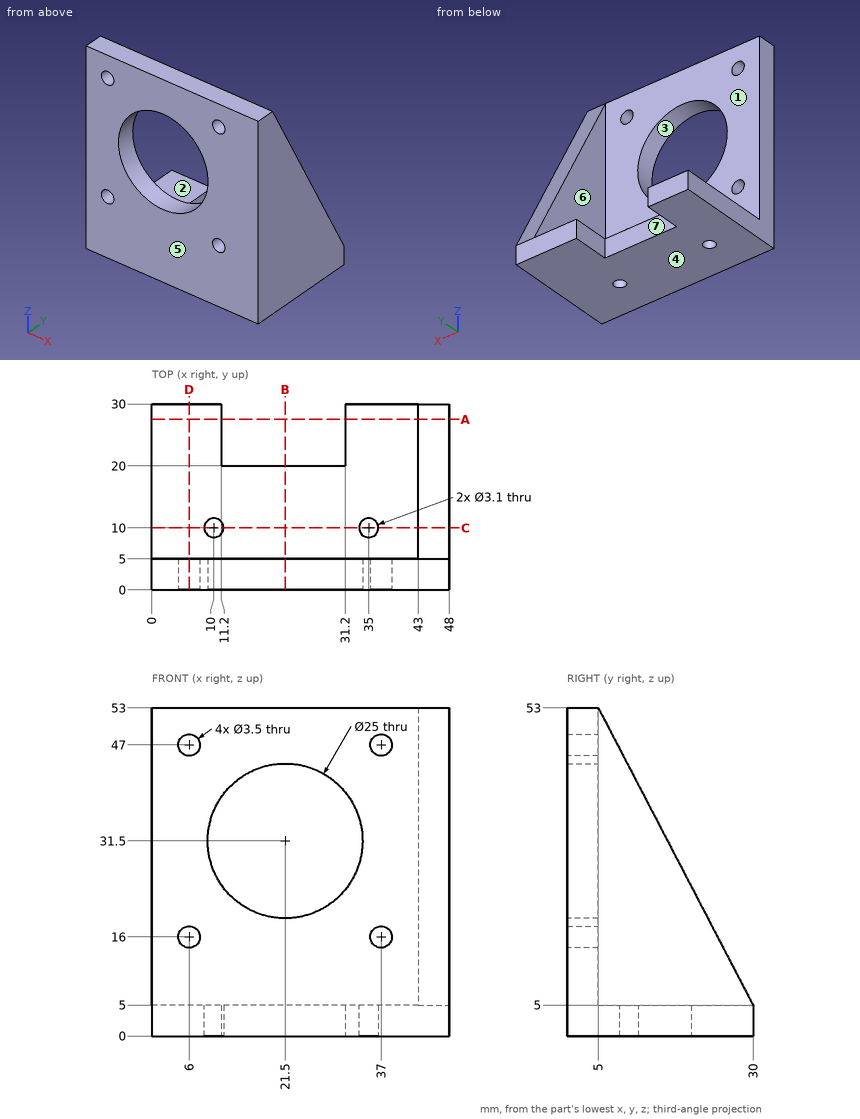
Input: dimensioned drawing with shaded views. Units: mm. Origin: part minimum x, y, z. A direction names the side the tool comes from. Coordinates: 2 decimals unless noted, no trailing zeros. Loops run counter-clockwise (first coordinate to the right, second up) from the corner with the lowest first, then second, coordinate; pieces in that order, holes last.
Q1. Section C-C, the plane y = 10. Return the cut outline in (x, z), and give its area (3 significant figures).
Results are:
outline: (0, 0) - (8.45, 0) - (8.45, 5) - (0, 5) - close; (11.55, 0) - (33.45, 0) - (33.45, 5) - (11.55, 5) - close; (36.55, 0) - (48, 0) - (48, 43.4) - (43, 43.4) - (43, 5) - (36.55, 5) - close
area: 401 mm2
Q2. Line query: line 1 along X through (y, z) = (2.3, 16); line 2 along Z through (x, y) = (21, 2); line 3 along Y through (x, z) = (35, 46). Output: solid intervals per line, ascending.
Results are:
line 1: x = 0 to 4.25, 7.75 to 35.25, 38.75 to 48
line 2: z = 0 to 19.01, 43.99 to 53
line 3: y = 0 to 5
Q3. Section B-B, the plane x = 21.5. Return the cut outline in (y, z).
Results are:
outline: (0, 0) - (20, 0) - (20, 5) - (5, 5) - (5, 19) - (0, 19) - close; (0, 44) - (5, 44) - (5, 53) - (0, 53) - close
Q4. Section D-D, the plane x = 6. Return the cut outline in (y, z).
Results are:
outline: (0, 0) - (30, 0) - (30, 5) - (5, 5) - (5, 14.25) - (0, 14.25) - close; (0, 17.75) - (5, 17.75) - (5, 45.25) - (0, 45.25) - close; (0, 48.75) - (5, 48.75) - (5, 53) - (0, 53) - close
Q5. Contact query for flat-ended pins moving along their axis: pin 1 (2 mm diameter, centred on x = 6, z = 47, fed in from -Y); pin 2 (4 mm diameter, centred on x = 23, z = 2.5, fed in from +Y); pin 3 (21.5 mm diameter, centred on x = 17, z = 29, fed in from +Y); pin 4 (7.5 mm diameter, centred on y = 15, z = 33.5, fed in from -X). Output: stop coordinate, or through.
Results are:
pin 1: passes through
pin 2: stops at y = 20
pin 3: stops at y = 5
pin 4: stops at x = 43
Q6. Mould query, pull axis Z, two halves, no side actions, for the marked faces 1, 2, 3 and 4. Classes: +Z half, -Z half, draft (parallel to the pull), parting line (faces both ways), or undercut.
Results are:
face 1: draft
face 2: +Z half
face 3: undercut
face 4: -Z half
Q7. Section A-A, the plane y = 27.5. Return the cut outline in (x, z).
Results are:
outline: (0, 0) - (11.2, 0) - (11.2, 5) - (0, 5) - close; (31.2, 0) - (48, 0) - (48, 9.8) - (43, 9.8) - (43, 5) - (31.2, 5) - close
Q8. Set-up query: the marked faces 5, 6 and 7. Return all of +Z, -Z, +X, -X, +Y, -Y with unobstructed straight access to the full face (end or side cutting, diameter ignored); none if empty.
Results are:
face 5: +Z, -Z, +X, -X, -Y
face 6: +Z, -X, +Y
face 7: +Z, -Z, +Y
